Source: CAD feature listing. Evaluate the final solid. Frame: model axes, mm. Face numbers are marked on the shaded views. A direction names the side the tool comes from. Round coordinates to 2 decimals unless told otherwise and drop trailing zeros. Loops run counter-clockwise (first coordinate to the right, second up) from the corner with the lowest first, then second, coordinate; pieces in that order, holes last. Notation, with made-up numbers: (-6, 54.5) - (34, 54.5) arc R16 cw to (34, 62.5) - close; hole circle Ø7 at (-9.5, 81.5). An arc over 180 degrees is marked (long way). Write item = value, one per line. Start each with the question number.
from build123d import *

# Parameters (mm, degrees)
F0_W     = 120
F0_H     = 120
F1_DEPTH = 6
F2_R     = 6
F3_W     = 5.722270757
F3_H     = 114
F4_DEPTH = 100
F5_R     = 2
F6_R     = 1.99999


# Not quite as in the source:
# - a fillet or chamfer is up to 0.001 mm smaller than in the source, because OpenCascade refuses the exact size


with BuildPart() as f1:
    # F0 (on Front) → F1 (new body)
    with BuildSketch(Plane.XZ):
        with Locations((3.6820918322, -11.3266304067)):
            Rectangle(F0_W, F0_H)
    extrude(amount=F1_DEPTH)

    # F2
    f2_edges = [f1.edges().sort_by_distance(p)[0] for p in [
        (-56.317908, -3, 48.67337),
    ]]
    fillet(f2_edges, radius=F2_R)

    # F3 (on face) → F4 (join)
    with BuildSketch(Plane.XZ.offset(6)):
        with Locations((-53.4567727894, -14.3266304067)):
            Rectangle(F3_W, F3_H)
    extrude(amount=F4_DEPTH)

    # F5
    f5_edges = [f1.edges().sort_by_distance(p)[0] for p in [
        (-56.317908, -56, 42.67337),
        (-50.595637, -56, 42.67337),
    ]]
    fillet(f5_edges, radius=F5_R)

    # F6 (radius 2 in the source; OpenCascade refuses exactly that, so slightly less here)
    f6_edges = [f1.edges().sort_by_distance(p)[0] for p in [
        (6.682092, -6, 48.67337),
        (6.682092, 0, 48.67337),
    ]]
    fillet(f6_edges, radius=F6_R)


solid = f1.part
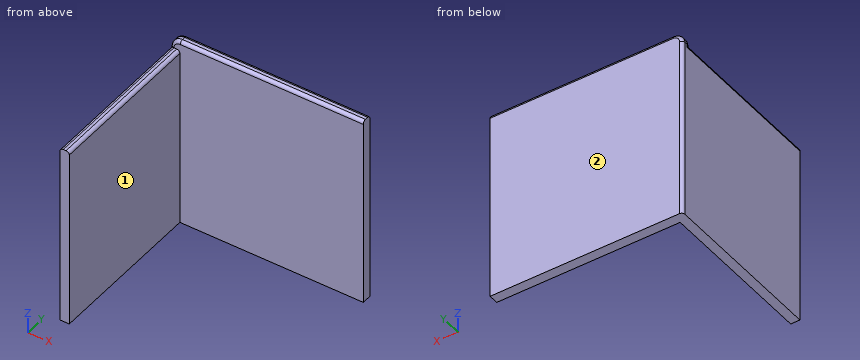
(1) Cut plane C-C (y = -43.5). Output: boundary loops of the cut face in (x, z), and give its area (3 significant figures).
(2) Material intervals for line 1 along Y through (x, z) = (38, 32); line 2 along X through (y, z) = (-57, -7.5); line 3 along Z through (x, y) = (56, -5.5), sorted ascending. Write a range as from..to.
(3) Cut plane B-B (x = -9). Output: boundary loops of the cut face in (y, z).
(4) Access query for the marked faces 1 and 2. Directions: +Z, -Z, +X, -X, +Y, -Y. A direction counts if a zero-diameter tool reaches every point of the face in a straight line with its end or side. Return the directions, or none.
(5) Cut plane A-A (z = -37.5). Output: boundary loops of the cut face in (x, y), and give its area (3 significant figures).
(6) Pin query (flat end, axial travel): P1, Ø8, axis at x = 24.5, z = -20, coming from the -Y side; P2, Ø4, axis at y = -95, z = -14.5, coming from the +X side; P3, Ø1.9, axis at x = -53.5, y = -75, coming from the +Z side. Return the tip coordinate at first contact, or that it passes through.
Solution:
q1.outline = (-56.32, -71.33) - (-50.6, -71.33) - (-50.6, 40.67) arc R2 ccw to (-52.6, 42.67) - (-54.32, 42.67) arc R2 ccw to (-56.32, 40.67) - close
q1.area = 651 mm^2
q2.line_1 = -6..0
q2.line_2 = -56.32..-50.6
q2.line_3 = -71.33..48
q3.outline = (-6, -71.33) - (0, -71.33) - (0, 46.67) arc R2 ccw to (-2, 48.67) - (-4, 48.67) arc R2 ccw to (-6, 46.67) - close
q4.face_1 = +Z, -Z, +X, -Y
q4.face_2 = +Z, -Z, +X, -X, +Y
q5.outline = (-56.32, -106) - (-50.6, -106) - (-50.6, -6) - (63.68, -6) - (63.68, 0) - (-54.32, 0) arc R2 ccw to (-56.32, -2) - close
q5.area = 1,290 mm^2
q6.P1 = -6
q6.P2 = -50.6
q6.P3 = 42.67
